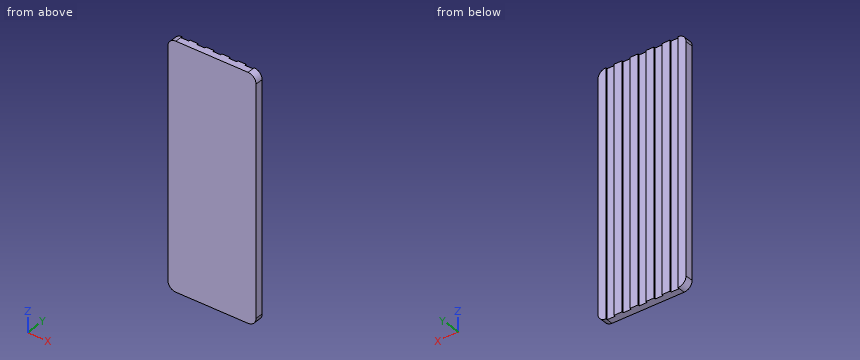
```python
from build123d import *

# Parameters (mm, degrees)
SKETCH2_W           = 55
SKETCH2_H           = 150
BOSS_EXTRUDE1_DEPTH = 5
FILLET1_R           = 5
SKETCH4_W           = 5
SKETCH4_H           = 1
CUT_EXTRUDE1_DEPTH  = 153.581945197
LPATTERN1_COUNT     = 5
LPATTERN1_PITCH     = 10


with BuildPart() as part:
    # Sketch2 → Boss-Extrude1 (new body)
    with BuildSketch(Plane(origin=(0, 0, 0), x_dir=(1, 0, 0), z_dir=(0, 1, 0))):
        Rectangle(SKETCH2_W, SKETCH2_H)
    extrude(amount=BOSS_EXTRUDE1_DEPTH)

    # Fillet1
    fillet1_edges = [part.edges().sort_by_distance(p)[0] for p in [
        (27.5, 2.5, 75),
        (-27.5, 2.5, 75),
        (-27.5, 2.5, -75),
        (27.5, 2.5, -75),
    ]]
    fillet(fillet1_edges, radius=FILLET1_R)

    # Sketch4 → Cut-Extrude1 (cut, through all)
    with BuildSketch(Plane.XY.offset(75)):
        with Locations((-20, 4.5)):
            Rectangle(SKETCH4_W, SKETCH4_H)
    cut_extrude1 = extrude(amount=-CUT_EXTRUDE1_DEPTH, mode=Mode.SUBTRACT)

    # LPattern1: Cut-Extrude1 ×5
    with Locations(*[(i * LPATTERN1_PITCH, 0, 0) for i in range(1, LPATTERN1_COUNT)]):
        add(cut_extrude1, mode=Mode.SUBTRACT)


solid = part.part
```
Build history of the part. All positions in model axes, mm. Coordinates: 2 decimals unless noted, no trailing zeros. Write each loop counter-clockwise with the first axis right and the second up, starting at its lowest first coordinate (ties: lowest second). Pieces come first, ordered by that corner, then holes.
1. Drill centre lines: probe 1 along X at (y, z) = (4.3, -43); probe 2 along Y at (x, z) = (-21, 51.5). Where is each one in solid material? Low to high.
Answer block:
probe 1: x = -27.5 to -22.5, -17.5 to -12.5, -7.5 to -2.5, 2.5 to 7.5, 12.5 to 17.5, 22.5 to 27.5
probe 2: y = 0 to 4
2. Drop a flat-ended pin along its axis: pin 1 (2.5 mm diameter, centred on x = -1, z = -6.5, fed in from +Y). Give the stop position or say it passes through.
Answer block:
pin 1: stops at y = 4
3. Band-saw the part on A-A, the plane z = 32.5. Give the cut face in (x, y), and give its area (3 significant figures).
Answer block:
outline: (-27.5, 0) - (27.5, 0) - (27.5, 5) - (22.5, 5) - (22.5, 4) - (17.5, 4) - (17.5, 5) - (12.5, 5) - (12.5, 4) - (7.5, 4) - (7.5, 5) - (2.5, 5) - (2.5, 4) - (-2.5, 4) - (-2.5, 5) - (-7.5, 5) - (-7.5, 4) - (-12.5, 4) - (-12.5, 5) - (-17.5, 5) - (-17.5, 4) - (-22.5, 4) - (-22.5, 5) - (-27.5, 5) - close
area: 250 mm2
